from build123d import *

# Parameters (mm, degrees)
F2_R     = 205.006654
F3_DEPTH = 350


with BuildPart() as f1:
    # F0 (on Front) → F1 (revolve)
    with BuildSketch(Plane.XZ):
        Polygon((30.885566, 166.75), (0, 166.75), (0, 100.9), (768.35, 100.9), (768.35, 187.6), (507.8, 187.6), (449.3, 129.1), (30.885566, 129.1), align=None)
    revolve(axis=Axis((384.175, 0, 0), (1, 0, 0)))

    # F2 (on face) → F3 (cut)
    with BuildSketch(Plane.YZ.offset(768.35)):
        Circle(F2_R)
        with BuildLine():
            ThreePointArc((187.6, 0), (-107.782791, -153.546833), (-63.75, 176.4361))
            Line((-63.75, 176.4361), (-63.75, 178.985858))
            ThreePointArc((-63.75, 178.985858), (0, 190), (63.75, 178.985858))
            Line((63.75, 178.985858), (63.75, 176.4361))
            ThreePointArc((63.75, 176.4361), (153.546833, 107.782791), (187.6, 0))
        make_face(mode=Mode.SUBTRACT)
        with BuildLine():
            ThreePointArc((63.75, 159.157281), (0, -171.45), (-63.75, 159.157281))
            Line((-63.75, 159.157281), (-63.75, 176.4361))
            ThreePointArc((-63.75, 176.4361), (-107.782791, -153.546833), (187.6, 0))
            ThreePointArc((187.6, 0), (153.546833, 107.782791), (63.75, 176.4361))
            Line((63.75, 176.4361), (63.75, 159.157281))
        make_face()
    extrude(amount=-F3_DEPTH, mode=Mode.SUBTRACT)


solid = f1.part
Part model, mm, in its own coordinate system. A direction names the side the tool comes from. Coordinates: 2 decimals unless noted, no trailing zeros. Loops run counter-clockwise (first coordinate to the right, second up) from the corner with the lowest first, then second, coordinate; pieces in that order, holes last. Notation, with made-up numbers: (33.25, 17) - (88.25, 17) arc R9 cw to (88.25, 34) - close; hole circle Ø6 at (41, 45). An arc over 180 degrees is marked (long way). Write each question's results on one line, items separated by ' | '. Start each with the question number.
Q1. Slice it at D-D on x = 404.5. Give the cut face in (y, z).
Q2. Slice it at B-B on z = 0. Give the cut face in (x, y).
Q3. Which spindle directions (+Z, -Z, +X, -X, +Y, -Y) get a long thin tool onto all of the face, cutting with end or side? Do faces 4 (the flat face through (768.35, -79, -69)), 5 (the flat face through (632, -63.75, 168)), 6 (the flat face through (30.886, 98, -86)), 7 (the flat face through (632, 63.75, 168)), 8 (the cylindrical face through (15.227, 162.785, -36.148)). Say none if no direction does.
Q4. Probe line 1 along Y through (x, z) = (316, 0); line 2 along Z through (x, y) = (555, 0); line 3 along Y through (x, z) = (584, 0). List the from-to ranges inside material, lowest first.
Q5. Slice it at A-A on y = 0. Give the cut face in (x, z).
Q6. Drop flat-ended pins along their axis: pin 1 Ø12 at (x, z) = (594, 119) entering from +Y; pin 2 Ø5 at (x, z) = (579, 170) entering from +Y; pin 3 Ø19 at (x, z) = (613, 167) entering from -Y. Give the stop position or say it passes through.
Q7. Slice it at C-C on x = 671. Give the cut face in (y, z), and give its area (3 significant figures).
Q8. Two-plate mould, pull along Y, no slides. Class faces 1 (the flat face through (0, 72, 72)), 2 (the cylindrical face through (636.251, 0.911, 187.598)), 3 (the cylindrical face through (389.55, -100.04, -13.14)): +Y half, -Y half, draft (parallel to the pull), parting line (faces both ways), or undercut.
Answer:
1) outline: circle Ø258.2 at (0, 0); hole circle Ø201.8 at (0, 0)
2) outline: (0, -166.75) - (30.89, -166.75) - (30.89, -129.1) - (449.3, -129.1) - (491.65, -171.45) - (768.35, -171.45) - (768.35, -100.9) - (0, -100.9) - close; (0, 100.9) - (768.35, 100.9) - (768.35, 171.45) - (491.65, 171.45) - (449.3, 129.1) - (30.89, 129.1) - (30.89, 166.75) - (0, 166.75) - close
3) face 4: +Z, -Z, +X, +Y, -Y | face 5: +Z, +X, -X, -Y | face 6: none | face 7: +Z, +X, -X, +Y | face 8: -X
4) line 1: y = -129.1 to -100.9, 100.9 to 129.1 | line 2: z = -171.45 to -100.9, 100.9 to 187.6 | line 3: y = -171.45 to -100.9, 100.9 to 171.45
5) outline: (0, -166.75) - (30.89, -166.75) - (30.89, -129.1) - (449.3, -129.1) - (491.65, -171.45) - (768.35, -171.45) - (768.35, -100.9) - (0, -100.9) - close; (0, 100.9) - (768.35, 100.9) - (768.35, 187.6) - (507.8, 187.6) - (449.3, 129.1) - (30.89, 129.1) - (30.89, 166.75) - (0, 166.75) - close
6) pin 1: stops at y = 128.94 | pin 2: stops at y = 63.75 | pin 3: stops at y = -67.74
7) outline: (-63.75, 159.16) arc R171.45 ccw (long way) to (63.75, 159.16) - (63.75, 176.44) arc R187.6 ccw to (-63.75, 176.44) - close; hole circle Ø201.8 at (0, 0) | area: 62,500 mm2
8) face 1: draft | face 2: parting line | face 3: undercut
